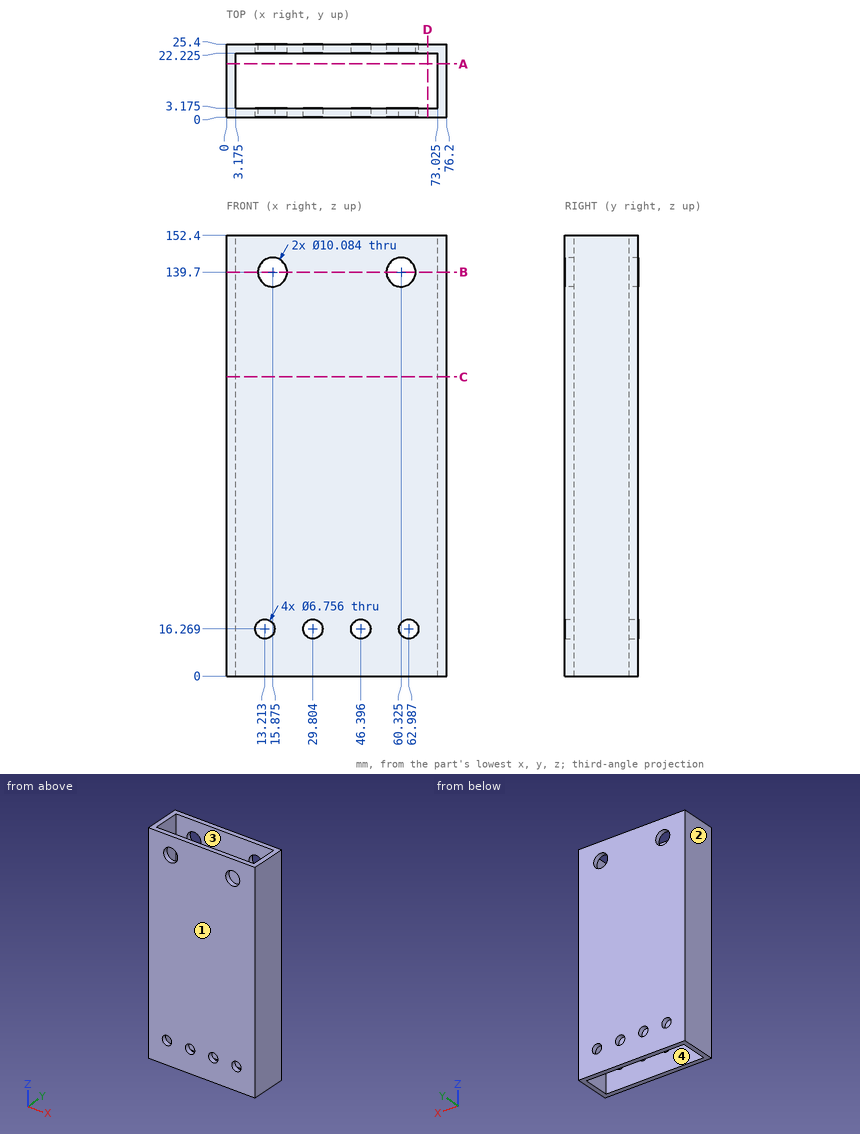
Check sheet for the drawn part. Datum: minimum x, y, z corner. Units: mm. Round coordinates to 2 decimals unless told otherwise and drop trailing zeros. Write each loop counter-clockwise with the first axis right and the second up, starting at its lowest first coordinate (ties: lowest second). Pieces come first, ordered by that corner, then holes. Notation, with made-up numbers: (36, 34.25) -> (92, 34.25) arc R10 ccw to (92, 46.25) -> close; hole circle Ø2 at (82.25, -2.75). An arc over 180 degrees is marked (long way). Put each result on its own line as item: value.
(1) Sectioned sample at C-C (z = 103.5). Enter the section's corners in (x, y) (1 decimal).
Values found:
outline: (0, 0) -> (76.2, 0) -> (76.2, 25.4) -> (0, 25.4) -> close; hole (3.2, 3.2) -> (73, 3.2) -> (73, 22.2) -> (3.2, 22.2) -> close
(2) Sectioned sample at A-A (y = 18.5). Enter the section's corners in (x, z) (1 decimal).
Values found:
outline: (0, 0) -> (3.2, 0) -> (3.2, 152.4) -> (0, 152.4) -> close; (73, 0) -> (76.2, 0) -> (76.2, 152.4) -> (73, 152.4) -> close
(3) Material ranges on line 1 (Y direction, x = 64, z = 97) (1 decimal); line 2 (X direction, y = 9.5, z = 52) (1 decimal); line 3 (X direction, y = 24.5, z = 143) (1 decimal), recorded low to high.
Values found:
line 1: y = 0 to 3.2, 22.2 to 25.4
line 2: x = 0 to 3.2, 73 to 76.2
line 3: x = 0 to 12.1, 19.7 to 56.5, 64.1 to 76.2
(4) Sectioned sample at D-D (x = 69.5). Enter the section's corners in (y, z) (1 decimal).
Values found:
outline: (0, 0) -> (3.2, 0) -> (3.2, 152.4) -> (0, 152.4) -> close; (22.2, 0) -> (25.4, 0) -> (25.4, 152.4) -> (22.2, 152.4) -> close
(5) Sectioned sample at B-B (z = 139.7). Enter the section's corners in (x, y) (1 decimal).
Values found:
outline: (0, 0) -> (10.8, 0) -> (10.8, 3.2) -> (3.2, 3.2) -> (3.2, 22.2) -> (10.8, 22.2) -> (10.8, 25.4) -> (0, 25.4) -> close; (20.9, 0) -> (55.3, 0) -> (55.3, 3.2) -> (20.9, 3.2) -> close; (20.9, 22.2) -> (55.3, 22.2) -> (55.3, 25.4) -> (20.9, 25.4) -> close; (65.4, 0) -> (76.2, 0) -> (76.2, 25.4) -> (65.4, 25.4) -> (65.4, 22.2) -> (73, 22.2) -> (73, 3.2) -> (65.4, 3.2) -> close
(6) Mould release check, pull along X, two halves, no side actions. Record for the marked faces 1, 2, 3 and 4: released by +X, released by -X, zero draft, split by the parting line, or undercut.
Values found:
face 1: zero draft
face 2: released by -X
face 3: undercut
face 4: undercut
